Here's how the part is built. I have some questions about the finished solid (model axes, mm). A direction names the side the tool comes from. Round coordinates to 2 decimals unless told otherwise and drop trailing zeros. Order: outer loops, then holes, each group sorted by start corner. A loop starts at its lowest first (then second) coordinate and runs counter-clockwise, first axis right, second up.
```python
from build123d import *

# Parameters (mm, degrees)
SKETCH_R     = 5.334
PAD_DEPTH    = 12.065
SKETCH001_R  = 8.89
PAD001_DEPTH = 2.286
SKETCH002_R  = 4.572
POCKET_DEPTH = 3.302
FILLET_R     = 2.032


with BuildPart() as part:
    # Sketch → Pad (new body)
    with BuildSketch(Plane.XY):
        Circle(SKETCH_R)
    extrude(amount=PAD_DEPTH)

    # Sketch001 → Pad001 (new body)
    with BuildSketch(Plane(origin=(0, 0, 0), x_dir=(1, 0, 0), z_dir=(0, 0, -1))):
        Circle(SKETCH001_R)
    extrude(amount=PAD001_DEPTH)

    # Sketch002 → Pocket (cut)
    with BuildSketch(Plane(origin=(0, 0, -2.286), x_dir=(1, 0, 0), z_dir=(0, 0, -1))):
        Circle(SKETCH002_R)
    extrude(amount=-POCKET_DEPTH, mode=Mode.SUBTRACT)

    # Fillet
    fillet_edges = [part.edges().sort_by_distance(p)[0] for p in [
        (-5.334, 0, 12.065),
    ]]
    fillet(fillet_edges, radius=FILLET_R)


solid = part.part
```
1) If we section it at A-A (y = 0): Write out the boundary of the cut face in (x, z) (3 decimals).
2) I need wall thicknesses on line 1 (Y direction, x = 0, z = -1.1); line 2 (Y direction, x = 0, z = 0.35). Which ranges of each line are inside material? Lowest first, please.
3) I'm going to push flat-ended pins straight in: pin 1 (3 mm diameter, centred on x = -4, z = 0.5, fed in from -Y); pin 2 (4 mm diameter, centred on x = -5.5, z = 2.5, fed in from -Y); pin 3 (6 mm diameter, centred on y = -1, z = 5, fed in from +X); pin 4 (1.5 mm diameter, centred on y = -7, z = 7, fed in from +X). Where does each tip first touch, or does it pass through?
4) For faces 4 (the cylindrical face through (-1.93, 8.68, -1.13)), 5 (the flat face through (4, 4, 0)), 6 (the cylindrical face through (-0.991, 4.463, -0.658)), which set-ups out of +Z, -Z, +X, -X, +Y, -Y let a thin tool reach every point of the face, with its end or its side?
5) We'd pull the mould along X, two halves only. Please class faces 1 (the cylindrical face through (2.461, -4.732, 4.946)), 2 (the flat face through (0, 0, 1.016)), 3 (the flat face through (0, 0, 12.065)): +X half, -X half, draft (parallel to the pull), parting line (faces both ways), or undercut.
6) If we section it at B-B (z = 0.75): Write out the boundary of the cut face in (x, y), plus the area to 3 significant figures.
7) If we section it at D-D (y = 6.25): Write out the boundary of the cut face in (x, z), plus the area to 3 significant figures.
Solutions:
1. outline: (-8.89, -2.286) - (-4.572, -2.286) - (-4.572, 1.016) - (4.572, 1.016) - (4.572, -2.286) - (8.89, -2.286) - (8.89, 0) - (5.334, 0) - (5.334, 10.033) arc R2.032 ccw to (3.302, 12.065) - (-3.302, 12.065) arc R2.032 ccw to (-5.334, 10.033) - (-5.334, 0) - (-8.89, 0) - close
2. line 1: y = -8.89 to -4.57, 4.57 to 8.89
2. line 2: y = -5.33 to -4.57, 4.57 to 5.33
3. pin 1: stops at y = -8.51
3. pin 2: stops at y = -4.03
3. pin 3: stops at x = 5.33
3. pin 4: passes through
4. face 4: +Z, -Z
4. face 5: +Z
4. face 6: -Z
5. face 1: parting line
5. face 2: undercut
5. face 3: draft
6. outline: circle Ø10.67 at (0, 0); hole circle Ø9.14 at (0, 0)
6. area: 23.7 mm2
7. outline: (-6.32, -2.29) - (6.32, -2.29) - (6.32, 0) - (-6.32, 0) - close
7. area: 28.9 mm2
